```python
from build123d import *

# Parameters (mm, degrees)
BOSS_EXTRUDE1_DEPTH = 391.865756272
SKETCH2_R           = 6.35
SKETCH2_R_2         = 14.2875
SKETCH2_R_3         = 2.0828
CUT_EXTRUDE1_DEPTH  = 141.732
SKETCH14_R          = 3.302
SKETCH14_W          = 25.4
SKETCH14_H          = 25.4
CUT_EXTRUDE12_DEPTH = 23.114
CUT_EXTRUDE13_DEPTH = 101.6


with BuildPart() as part:
    # Sketch1 → Boss-Extrude1 (new body, symmetric)
    with BuildSketch(Plane(origin=(0, 0, 0), x_dir=(0, 0, -1), z_dir=(1, 0, 0))):
        Polygon((-38.1, 50.8), (38.1, 50.8), (38.1, -50.8), (34.925, -50.8), (34.925, 47.625), (-34.925, 47.625), (-34.925, -50.8), (-38.1, -50.8), align=None)
    extrude(amount=BOSS_EXTRUDE1_DEPTH, both=True)

    # Sketch2 → Cut-Extrude1 (cut)
    with BuildSketch(Plane.XY.offset(38.1)):
        with Locations((-341.065756187, -7.9375)):
            Circle(SKETCH2_R)
        with Locations((122.51182, -33.3375)):
            Circle(SKETCH2_R_2)
        with Locations((341.065756187, -7.9375)):
            Circle(SKETCH2_R)
        with Locations((12.7, 34.925)):
            Circle(SKETCH2_R_3)
        with Locations((-279.4, 34.925)):
            Circle(SKETCH2_R_3)
        with Locations((-122.51182, -33.3375)):
            Circle(SKETCH2_R_2)
    extrude(amount=-CUT_EXTRUDE1_DEPTH, mode=Mode.SUBTRACT)

    # Sketch14 → Cut-Extrude12 (cut)
    with BuildSketch(Plane(origin=(0, 0, -38.1), x_dir=(-1, 0, 0), z_dir=(0, 0, -1))):
        with Locations((-160.61182, -35.123476108)):
            Circle(SKETCH14_R)
        with Locations((-160.61182, 41.076523892)):
            Circle(SKETCH14_R)
        with Locations((-84.41182, 41.076523892)):
            Circle(SKETCH14_R)
        with Locations((-84.41182, -35.123476108)):
            Circle(SKETCH14_R)
        with Locations((-12.7, 34.925)):
            Rectangle(SKETCH14_W, SKETCH14_H)
        with Locations((279.4, 34.925)):
            Rectangle(SKETCH14_W, SKETCH14_H)
    extrude(amount=-CUT_EXTRUDE12_DEPTH, mode=Mode.SUBTRACT)

    # Sketch16 → Cut-Extrude13 (cut)
    with BuildSketch(Plane.XY.offset(38.1)):
        Polygon((-391.865756272, 25.4), (-347.87166576, -50.8), (-391.865756272, -50.8), align=None)
        Polygon((347.87166576, -50.8), (391.865756272, -50.8), (391.865756272, 25.4), align=None)
    extrude(amount=-CUT_EXTRUDE13_DEPTH, mode=Mode.SUBTRACT)


solid = part.part
```
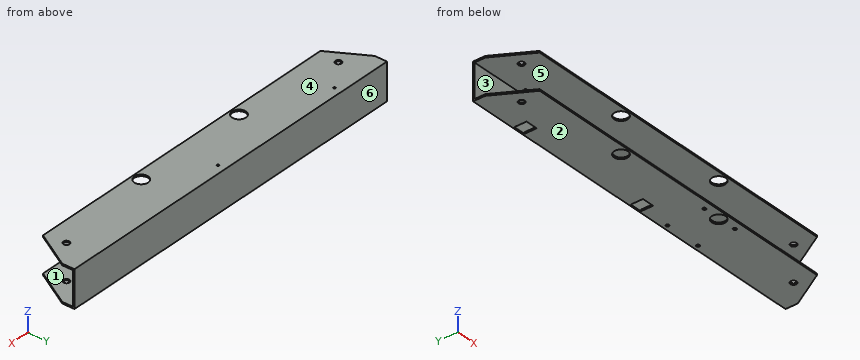
Geometry: final body of the model. Coordinates: model frame, mm. Face numbers are marked on the shaded views. A direction names the side the tool comes from. Round coordinates to 2 decimals unless told otherwise and drop trailing zeros. Write each loop counter-clockwise with the first axis right and the second up, starting at its lowest first coordinate (ties: lowest second). Pieces come first, ordered by that corner, then holes. Notation, with made-up numbers: M 72.25,-34.5 L 92.25,-34.5 A23 cw 92.25,-12.5 Z; hole C 55,89.25 d7. An arc over 180 degrees is marked long. Answer in a Markdown table with one row per item. Add a question column.
(1) Cut plane B-B, the plane x = 212.5. Return the cut outline in (y, z) (3 decimals).
(2) Ray query, L1, parallel to Z at x = -98, y = -41.5 (3 decimals); L2, parallel to Y at x = -320, z = 1.5 (3 decimals). Return the intervals inside material, ascending.
(3) Cut plane C-C, the plane z = 27. Return the cut outline in (x, y) (3 decimals), then the cut area to 3 significant figures.
(4) Cut plane A-A, the plane y = 6. Return the cut outline in (x, z) (3 decimals), then the cut area to 3 significant figures.
(5) Reachability of the marked faces 1 and 2 from +Z, -Z, +X, -X, +Y, -Y: full face, straight path, thin tool, end or side. Return the list, or none.
(6) Contact query for flat-ended pins moving along their axis: pin 1 (5.5 mm diameter, centred on x = 84.41, y = 41.08, fed in from -Z) (3 decimals); pin 2 (6 mm diameter, centred on x = 143.5, z = 12.5, fed in from -Y) (3 decimals); pin 3 (6.5 mm diameter, centred on x = -279.4, y = 34.925, fed in from +Z). Output: stop coordinate, or through.
(7) Draft query along Z for the marked faces 3, 4, 5 and 6. Return one class per face: pulls with the +Z half, pulls with the -Z half, needs draft (parallel to the pull), parting line crosses it, or undercut.
Established:
| question | item | result |
|---|---|---|
| 1 | outline | M -50.8,-38.1 L 50.8,-38.1 L 50.8,38.1 L -50.8,38.1 L -50.8,34.925 L 47.625,34.925 L 47.625,-34.925 L -50.8,-34.925 Z |
| 2 | L1 | -38.1 to -34.925, 34.925 to 38.1 |
| 2 | L2 | 47.625 to 50.8 |
| 3 | outline | M -391.866,47.625 L 391.866,47.625 L 391.866,50.8 L -391.866,50.8 Z |
| 3 | area | 2,490 mm² |
| 4 | outline | M -380.665,-38.1 L 380.665,-38.1 L 380.665,-34.925 L -380.665,-34.925 Z; M -380.665,34.925 L 380.665,34.925 L 380.665,38.1 L -380.665,38.1 Z |
| 4 | area | 4,830 mm² |
| 5 | face 1 | +X, -X, -Y |
| 5 | face 2 | -Z, +X, -X, +Y, -Y |
| 6 | pin 1 | z = 34.925 |
| 6 | pin 2 | y = 47.625 |
| 6 | pin 3 | z = 38.1 |
| 7 | face 3 | undercut |
| 7 | face 4 | pulls with the +Z half |
| 7 | face 5 | undercut |
| 7 | face 6 | needs draft |
